The model under review builds one solid part; all positions refer to its coordinate system, in mm. Round coordinates to 2 decimals unless told otherwise and drop trailing zeros. Return JSON: item names as keys, results as strings.
from build123d import *

# Parameters (mm, degrees)
SKETCH1_R           = 80
BOSS_EXTRUDE1_DEPTH = 5
SKETCH2_R           = 4
SKETCH2_W           = 10
SKETCH2_H           = 20
CUT_EXTRUDE1_DEPTH  = 5
CIRPATTERN1_COUNT   = 18
SKETCH3_R           = 1.6
CUT_EXTRUDE2_DEPTH  = 5
SKETCH4_R           = 1.6
CUT_EXTRUDE3_DEPTH  = 10


with BuildPart() as part:
    # Sketch1 → Boss-Extrude1 (new body)
    with BuildSketch(Plane.XY):
        Circle(SKETCH1_R)
    extrude(amount=BOSS_EXTRUDE1_DEPTH)

    # Sketch2 → Cut-Extrude1 (cut)
    with BuildSketch(Plane.XY.offset(5)):
        Circle(SKETCH2_R)
        with Locations((0, 60)):
            Rectangle(SKETCH2_W, SKETCH2_H)
    cut_extrude1 = extrude(amount=-CUT_EXTRUDE1_DEPTH, mode=Mode.SUBTRACT)

    # CirPattern1: Cut-Extrude1 ×18 about axis
    cirpattern1_axis = Axis((0, 0, 0), (0, 0, 1))
    for i in range(1, CIRPATTERN1_COUNT):
        add(cut_extrude1.rotate(cirpattern1_axis, i * 360 / CIRPATTERN1_COUNT), mode=Mode.SUBTRACT)

    # Sketch3 → Cut-Extrude2 (cut)
    with BuildSketch(Plane.XY.offset(5)):
        with Locations((-55.155199905, 46.280707897)):
            Circle(SKETCH3_R)
        with Locations((-55.155199905, -46.280707897)):
            Circle(SKETCH3_R)
        with Locations((55.155199905, -46.280707897)):
            Circle(SKETCH3_R)
        with Locations((55.155199905, 46.280707897)):
            Circle(SKETCH3_R)
        with Locations((-40, 0)):
            Circle(SKETCH3_R)
        with Locations((0, 40)):
            Circle(SKETCH3_R)
        with Locations((0, -40)):
            Circle(SKETCH3_R)
        with Locations((40, 0)):
            Circle(SKETCH3_R)
    extrude(amount=-CUT_EXTRUDE2_DEPTH, mode=Mode.SUBTRACT)

    # Sketch4 → Cut-Extrude3 (cut)
    with BuildSketch(Plane(origin=(0, 0, 0), x_dir=(-1, 0, 0), z_dir=(0, 0, -1))):
        with Locations((-11.570176974, 13.788799976)):
            Circle(SKETCH4_R)
        with Locations((13.788799976, 11.570176974)):
            Circle(SKETCH4_R)
        with Locations((11.570176974, -13.788799976)):
            Circle(SKETCH4_R)
        with Locations((-13.788799976, -11.570176974)):
            Circle(SKETCH4_R)
    extrude(amount=-CUT_EXTRUDE3_DEPTH, mode=Mode.SUBTRACT)


solid = part.part
(1) Wall thickness on line 1 (Y direction, x = 0, z = 1.6); line 2 (Y direction, x = 57, z = 1.1); line 3 (Y direction, x = 65.5, z = 3.95): over which ranges is each line inside the solid? List them lowest first.
Filled in:
{"line 1": "y = -80 to -70, -50 to -41.6, -38.4 to -4, 4 to 38.4, 41.6 to 50, 70 to 80", "line 2": "y = -56.13 to -38.68, -27.14 to -15.13, -4.97 to 4.97, 15.13 to 27.14, 38.68 to 56.13", "line 3": "y = -45.93 to -16.63, -6.47 to 6.47, 16.63 to 45.93"}
(2) Mouldability with a two-part tool opening along Y and no side actions: class faces 1 (the flat face through (-32.19, 38.26, 2.54)), 2 (the cylindrical face through (-17.34, -78.1, 2.46)) as released by +Y, released by -Y, zero draft, split by the parting line, or undercut.
Filled in:
{"face 1": "undercut", "face 2": "split by the parting line"}
(3) Clearance check with flat-ended pins moving along their axes: pin 1 Ø1.9 at (x, y) = (0, -40) entering from +Z; pin 2 Ø1.5 at (y, z) = (55.5, 3) entering from -X; pin 3 Ø2.5 at (x, z) = (-2, 2) entering from +Y. State where each tip first meets the part, or that it passes through.
Filled in:
{"pin 1": "passes through", "pin 2": "stops at x = -58.33", "pin 3": "stops at y = 80"}
(4) Add section A-A (z = 2.4). Give the number of separate pieces and of enclosed holes in the cut face, plus the area to 3 significant figures.
Filled in:
{"separate pieces": "1", "enclosed holes": "31", "area": "16,400 mm2"}
